The figure shows three views and two pictorial views of one solid part (mm, origin at its lowest corner). Answer the questions. A direction names the side the tool comes from. Coordinates: 2 decimals unless noted, no trailing zeros. Order: outer loops, then holes, each group sorted by start corner. A loop starts at its lowest first (then second) coordinate and runs counter-clockwise, first axis right, second up.
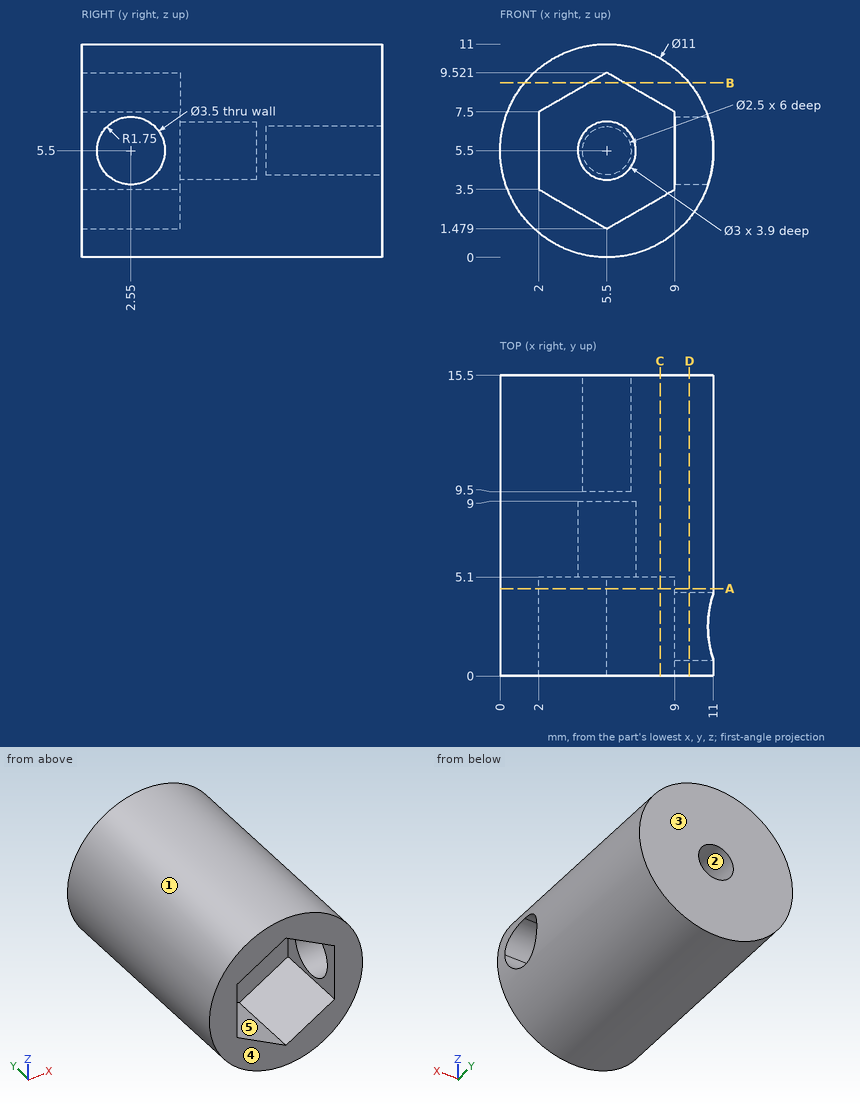
1) A cutting plane is placed at C-C, the plane x = 8.25. Write down the section's boundary in (y, z), plus the area to 3 significant figures.
2) Straight lines are drawn through the part: probe 1 along X at (y, z) = (6.8, 5.5); probe 2 along X at (y, z) = (11.75, 5.5); probe 3 along Y at (x, z) = (5, 4.75). For each, find the intervals that lie inside material, in ascending order.
3) A cutting plane is placed at D-D, the plane x = 9.75. Write down the section's boundary in (y, z).
4) A cutting plane is placed at B-B, the plane z = 9. Write down the section's boundary in (x, y), plus the area to 3 significant figures.
5) A cutting plane is placed at A-A, the plane y = 4.5. Write down the section's boundary in (x, z), plus the area to 3 significant figures.
6) Each of these flat-tipped pins is pushed along its axis until it touches: P1, Ø2, axis at x = 4.5, z = 4, coming from the -Y side; P2, Ø2, axis at y = 6.5, z = 9, coming from the -X side; P3, Ø0.8, axis at x = 5, z = 5.5, coming from the +Y side. Where does it stop, or does it pass through?
7) The mould has two halves that part along X. Classify the marked faces 1, 2 and 3: released by +X, released by -X, zero draft, split by the parting line, or undercut.
8) For the marked faces 4 and 5, determine the directions among +Z, -Z, +X, -X, +Y, -Y from which every point of the face is accessible in a straight line to the end or side of a thin tool.
Working result:
1. outline: (0, 0.74) - (15.5, 0.74) - (15.5, 10.26) - (0, 10.26) - (0, 7.93) - (5.1, 7.93) - (5.1, 3.07) - (0, 3.07) - close
1. area: 123 mm2
2. probe 1: x = 0 to 4, 7 to 11
2. probe 2: x = 0 to 4.25, 6.75 to 11
2. probe 3: y = 9 to 9.5
3. outline: (0, 2.01) - (15.5, 2.01) - (15.5, 8.99) - (0, 8.99) - close; hole circle Ø3.5 at (2.55, 5.5)
4. outline: (1.26, 0) - (4.6, 0) - (4.6, 5.1) - (6.4, 5.1) - (6.4, 0) - (9.74, 0) - (9.74, 15.5) - (1.26, 15.5) - close
4. area: 122 mm2
5. outline: circle Ø11 at (5.5, 5.5); hole (2, 3.5) - (5.5, 1.48) - (9, 3.5) - (9, 7.5) - (5.5, 9.52) - (2, 7.5) - close
5. area: 52.9 mm2
6. P1: stops at y = 5.1
6. P2: stops at x = 0.6
6. P3: stops at y = 9.5
7. face 1: split by the parting line
7. face 2: undercut
7. face 3: zero draft
8. face 4: +Z, -Z, +X, -X, -Y
8. face 5: -Y
